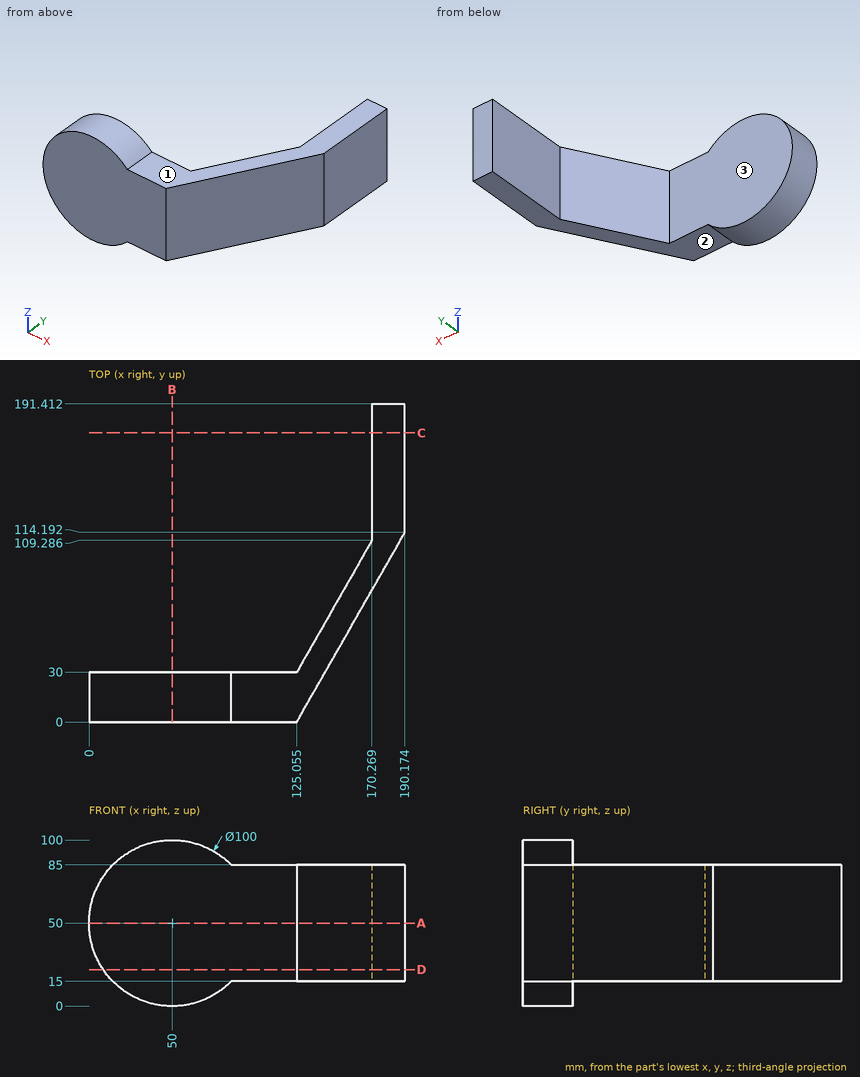
Design review of the part shown in the three views and the two pictorial views. Dimensions are in mm from the part's minimum x, y and z. A direction names the side the tool comes from. Coordinates: 2 decimals unless noted, no trailing zeros. Write each loop counter-clockwise with the first axis right and the second up, starting at its lowest first coordinate (ties: lowest second). Pieces come first, ordered by that corner, then holes.
(1) Add section C-C on y = 174. Give the boundary of the cut face in (x, z) (1 decimal), then the cut area to 3 significant figures.
(2) Add section D-D on z = 22. Give the boundary of the cut face in (x, y) (1 decimal).
(3) Wall thickness on probe 1 along X at (y, z) = (174.5, 34.5) (1 decimal); probe 2 along Y at (x, z) = (60, 41); probe 3 along Z at (x, y) = (123, 27.5): over which ranges is each line inside the solid? List them lowest first.
(4) For pin 1 Ø6 at (x, z) = (131.5, 21) entering from -Y; pin 2 Ø3 at (x, z) = (64, 73) entering from +Y, all flat-tipped, find the tip position at first contact; note any pin that passes through.
(5) Add section A-A on z = 50. Give the boundary of the cut face in (x, y) (1 decimal).
(6) Add section B-B on x = 50. Give the boundary of the cut face in (y, z).
(7) Tool access review of the marked faces 1, 2 and 3: name each direction out of +Z, -Z, +X, -X, +Y, -Y from which nothing blocks a thin tool from reaching the whole face with its end or side.
Answer sheet:
1. outline: (170.3, 15) - (190.2, 15) - (190.2, 85) - (170.3, 85) - close
1. area: 1,390 mm2
2. outline: (8.6, 0) - (125.1, 0) - (190.2, 114.2) - (190.2, 191.4) - (170.3, 191.4) - (170.3, 109.3) - (125.1, 30) - (8.6, 30) - close
3. probe 1: x = 170.3 to 190.2
3. probe 2: y = 0 to 30
3. probe 3: z = 15 to 85
4. pin 1: stops at y = 6.04
4. pin 2: stops at y = 30
5. outline: (0, 0) - (125.1, 0) - (190.2, 114.2) - (190.2, 191.4) - (170.3, 191.4) - (170.3, 109.3) - (125.1, 30) - (0, 30) - close
6. outline: (0, 0) - (30, 0) - (30, 100) - (0, 100) - close
7. face 1: +Z, +X, +Y, -Y
7. face 2: -Z, +X, +Y, -Y
7. face 3: +Z, -Z, -X, +Y
